The listing builds one solid part. Answer for the finished solid, in the listing's coordinates (mm). A direction names the side the tool comes from. Coordinates: 2 decimals unless noted, no trailing zeros. Loops run counter-clockwise (first coordinate to the right, second up) from the corner with the lowest first, then second, coordinate; pieces in that order, holes last. Notation, with made-up numbers: (51.25, 67.5) -> (68.25, 67.5) arc R29 cw to (68.25, 91.5) -> close; hole circle Ø11 at (20.25, -14.5). An arc over 180 degrees is marked (long way). Answer in a Markdown table with one row per item.
Autodesk Inventor part; units mm, degrees
ref_plane "YZ Plane" through (0, 0, 0) normal (1, 0, 0) x (0, 1, 0)
ref_plane "XZ Plane" through (0, 0, 0) normal (0, 1, 0) x (-1, 0, 0)
ref_plane "XY Plane" through (0, 0, 0) normal (0, 0, 1) x (1, 0, 0)
sketch "Sketch1" plane through (0, 0, 0) normal (0, 0, 1) x (1, 0, 0)
  line L0 (-16.75, 305) -> (16.75, 305)
  line L1 (16.75, 305) -> (16.75, 0)
  line L2 (16.75, 0) -> (-16.75, 0)
  line L3 (-16.75, 0) -> (-16.75, 305)
  point P0 (0, 0)
  point P1 (0, 0)
  point P2 (0, 0)
  point P3 (0, 0)
  point P4 (0, 0)
  dimension "d27" = 33.5
  dimension "d29" = 305
extrude "Plate1" add sketch "Sketch1" against normal blind 2
sketch "Sketch2" plane through (14.75, 305, -2) normal (1, 0, 0) x (0, 1, 0)
  line L0 (-305, 0) -> (0, 0)
  line L1 (0, 0) -> (0, 25)
  line L2 (0, 25) -> (-305, 25)
  line L3 (-305, 25) -> (-305, 0)
edge flange "Flange1" height 25 angle 90 thickness 2 bend radius 2 thickness toward (1, 0, 0) relief tear relief width 2 relief depth 1 corner gap 2 corner form 0 edges at (16.75, 152.5, 0) (-16.75, 152.5, 0) wall of the first edge with corners at (14.75, 0, -2) (14.75, 305, -2) (14.75, 305, 23) (14.75, 0, 23)
bend "Bend1"
corner "Corner1"
sketch "Sketch3" plane through (16.75, 0, 23) normal (1, 0, 0) x (0, 0, -1)
  line L0 (0, 305) -> (21, 305)
  line L1 (21, 305) -> (21, 0)
  line L2 (21, 305) -> (21, 310)
  line L3 (21, 310) -> (0, 310)
  line L4 (0, 310) -> (0, 305)
  point P0 (23, 0)
  dimension "d40" = 5
sheet face with bend "Face2" sketch "Sketch3" thickness 2 toward (-1, 0, 0) bend radius 2
bend "Bend2"
mirror "Mirror1" about plane through (0, 0, 0) normal (1, 0, 0)
sketch "Sketch4" plane through (16.75, 0, 23) normal (1, 0, 0) x (0, 0, -1)
  line L0 (0, 310) -> (0, 0)
  line L1 (0, 19.8595) -> (25, 15)
  line L2 (25, 305) -> (25, 0)
  line L3 (25, 0) -> (0, 0)
  line L4 (21, 310) -> (0, 310)
  point P0 (23, 0)
  dimension "d46" = 295
  dimension "d47" = 11
extrude "Extrusion1" cut sketch "Sketch4" along normal through all both and the other way through all
equation "\"d47\" = wheel_pin_Angle"
equation "\"d15\" = Thickness"
equation "\"d30\" = BendReliefWidth"
equation "\"d31\" = BendReliefDepth"
equation "\"d32\" = MinimumRemnant"
equation "\"d33\" = TransitionRadius"
equation "\"d34\" = wheel_pin_h"
equation "\"d36\" = BendRadius"
equation "\"d37\" = CornerReliefSize"
equation "\"d38\" = GapSize"
equation "\"d39\" = JacobiRadiusSize"
equation "\"GapSize\" = Thickness"
equation "\"BendRadius\" = Thickness"
equation "\"MinimumRemnant\" = 2 * Thickness"
equation "\"BendReliefDepth\" = 0.5 * Thickness"
equation "\"BendReliefWidth\" = Thickness"
equation "\"CornerReliefSize\" = 4 * Thickness"
equation "\"JacobiRadiusSize\" = BendRadius"
equation "\"TransitionRadius\" = BendRadius"
equation "\"d41\" = BendRadius"
equation "\"d42\" = BendReliefWidth"
equation "\"d44\" = MinimumRemnant"
equation "\"d43\" = BendReliefDepth"
equation "\"d45\" = TransitionRadius"
properties part number "DMF v2.1 gear wheel pin 1"
Item 1: Find the intervals of material crossed by probe 1 along X at (y, z) = (121, 15.25); probe 2 along Z at (x, y) = (6, 291); probe 3 along Y at (x, z) = (0.5, -0.25), in increasing order.
Findings below:
| item | result |
|---|---|
| probe 1 | x = -16.75 to -14.75, 14.75 to 16.75 |
| probe 2 | z = -2 to 0 |
| probe 3 | y = 15.34 to 305 |
Item 2: A cutting plane is placed at A-A, the plane y = 88.5. Determine the outline of the cut face in (x, z).
Findings below:
| item | result |
|---|---|
| outline | (-16.75, 2) arc R4 ccw to (-12.75, -2) -> (12.75, -2) arc R4 ccw to (16.75, 2) -> (16.75, 23) -> (14.75, 23) -> (14.75, 2) arc R2 cw to (12.75, 0) -> (-12.75, 0) arc R2 cw to (-14.75, 2) -> (-14.75, 23) -> (-16.75, 23) -> close |
Item 3: Determine the mould class of faces 1 (the face through (-16.75, 161, 13)), 2 (the face through (14.75, 165, 13)), 3 (the face through (16.75, 165, 13)) for opening direction X: +X half, -X half, draft (parallel to the pull), parting line (faces both ways), or undercut.
Findings below:
| item | result |
|---|---|
| face 1 | -X half |
| face 2 | undercut |
| face 3 | +X half |
Item 4: A cutting plane is placed at B-B, the plane z = 16.25. Determine the outline of the cut face in (x, y).
Findings below:
| item | result |
|---|---|
| outline | (-16.75, 18.55) -> (-14.75, 18.55) -> (-14.75, 310) -> (-16.75, 310) -> close; (14.75, 18.55) -> (16.75, 18.55) -> (16.75, 310) -> (14.75, 310) -> close |
Item 5: Flat-ended cylindrical pins translate along their axes: pin 1 Ø3 at (x, z) = (-5, -0.5) entering from +Y; pin 2 Ø7.5 at (x, y) = (0, 143) entering from +Z; pin 3 Ø1 at (x, y) = (-16, 307.5) entering from -Z. Find the tip coordinate at first contact, or state that the pin passes through.
Findings below:
| item | result |
|---|---|
| pin 1 | stops at y = 305 |
| pin 2 | stops at z = 0 |
| pin 3 | stops at z = 2 |
Item 6: A cutting plane is placed at C-C, the plane x = 10. Determine the outline of the cut face in (y, z).
Findings below:
| item | result |
|---|---|
| outline | (15, -2) -> (305, -2) -> (305, 0) -> (15.39, 0) -> close |
Item 7: A cutting plane is placed at D-D, the plane z = 4.5. Determine the outline of the cut face in (x, y).
Findings below:
| item | result |
|---|---|
| outline | (-16.75, 16.26) -> (-14.75, 16.26) -> (-14.75, 310) -> (-16.75, 310) -> close; (14.75, 16.26) -> (16.75, 16.26) -> (16.75, 310) -> (14.75, 310) -> close |
Item 8: A tool of negligible diameter and unlimited length cuts with its end or side. For faces 4 (the face through (0, 162, 0)), 5 (the face through (-0.08, 15.28, -0.55)), from which of +Z, -Z, +X, -X, +Y, -Y can it reach the whole face along a straight path? Write none if from no direction.
Findings below:
| item | result |
|---|---|
| face 4 | +Z, +Y, -Y |
| face 5 | +Z, +X, -X, -Y |
